Read the model definition and answer for the solid it produces. Units are mm, in the model's axes. Coordinates: 2 decimals unless noted, no trailing zeros. Write each loop counter-clockwise with the first axis right and the second up, starting at its lowest first coordinate (ties: lowest second). Pieces come first, ordered by that corner, then holes. Notation, with made-up numbers: (67.25, -20) -> (73.25, -20) arc R32 ccw to (73.25, 7) -> close; hole circle Ø11 at (-1.5, 9.25). An arc over 180 degrees is marked (long way). One line per item, written item: value. Start each with the question number.
1. Find section C-C, the plane y = 41.5. Write down the section's boundary in (x, z) (3 decimals).
2. Find section A-A, the plane y = -15.5. Write down the section's boundary in (x, z), and give its area (3 significant figures).
3. Given P1, Ø4, axis at x = -90, y = -41.5, coming from the -Z side, flat-ended and moving along its own axis, determine where the tip first touches the part or whether it passes through.
4. Consider line 1 along Y through (x, z) = (-90, 3.75) (3 decimals); line 2 along Y through (x, z) = (36, 6.75); line 3 along X through (y, z) = (21.5, 3.25). Determine where each line is inside the solid, lowest interval first.
5. Find section D-D, the plane z = 5.75. State how many separate pieces and enclosed holes the cut face has, and give its area (3 significant figures).
6. Find section B-B, the plane x = -71. Write down the section's boundary in (y, z), and give its area (3 significant figures).
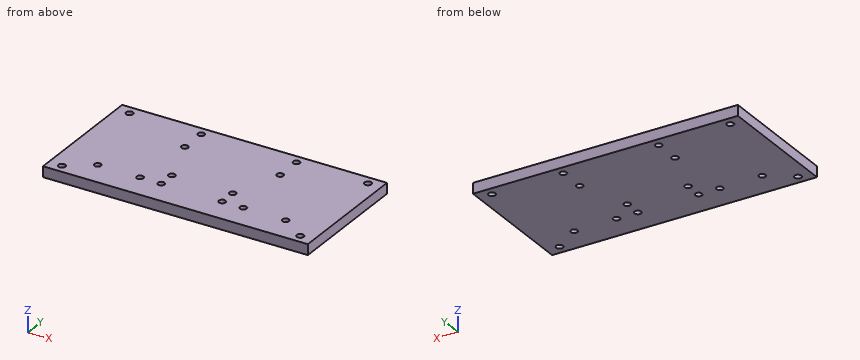
```python
from build123d import *

# Parameters (mm, degrees)
SKETCH_W   = 97
SKETCH_H   = 200
SKETCH_R   = 2.5
SKETCH_R_2 = 2.625
PAD_DEPTH  = 8


with BuildPart() as part:
    # Sketch → Pad (new body)
    with BuildSketch(Plane(origin=(0, 0, 0), x_dir=(0, 1, 0), z_dir=(0, 0, 1))):
        Rectangle(SKETCH_W, SKETCH_H)
        with Locations((-28.5, 71)):
            Circle(SKETCH_R, mode=Mode.SUBTRACT)
        with Locations((-28.5, 39)):
            Circle(SKETCH_R, mode=Mode.SUBTRACT)
        with Locations((-28.5, -39)):
            Circle(SKETCH_R, mode=Mode.SUBTRACT)
        with Locations((-28.5, -71)):
            Circle(SKETCH_R, mode=Mode.SUBTRACT)
        with Locations((-28.5, 23)):
            Circle(SKETCH_R, mode=Mode.SUBTRACT)
        with Locations((-15.5, 23)):
            Circle(SKETCH_R, mode=Mode.SUBTRACT)
        with Locations((-28.5, -23)):
            Circle(SKETCH_R, mode=Mode.SUBTRACT)
        with Locations((-15.5, -23)):
            Circle(SKETCH_R, mode=Mode.SUBTRACT)
        with Locations((-41.5, 90)):
            Circle(SKETCH_R_2, mode=Mode.SUBTRACT)
        with Locations((41.5, 90)):
            Circle(SKETCH_R_2, mode=Mode.SUBTRACT)
        with Locations((-41.5, -90)):
            Circle(SKETCH_R_2, mode=Mode.SUBTRACT)
        with Locations((41.5, -90)):
            Circle(SKETCH_R_2, mode=Mode.SUBTRACT)
        with Locations((21.5, 36)):
            Circle(SKETCH_R, mode=Mode.SUBTRACT)
        with Locations((41.5, 36)):
            Circle(SKETCH_R, mode=Mode.SUBTRACT)
        with Locations((21.5, -36)):
            Circle(SKETCH_R, mode=Mode.SUBTRACT)
        with Locations((41.5, -36)):
            Circle(SKETCH_R, mode=Mode.SUBTRACT)
    extrude(amount=PAD_DEPTH)


solid = part.part
```
Answer block:
1. outline: (-100, 0) -> (-92.625, 0) -> (-92.625, 8) -> (-100, 8) -> close; (-87.375, 0) -> (-38.5, 0) -> (-38.5, 8) -> (-87.375, 8) -> close; (-33.5, 0) -> (33.5, 0) -> (33.5, 8) -> (-33.5, 8) -> close; (38.5, 0) -> (87.375, 0) -> (87.375, 8) -> (38.5, 8) -> close; (92.625, 0) -> (100, 0) -> (100, 8) -> (92.625, 8) -> close
2. outline: (-100, 0) -> (-25.5, 0) -> (-25.5, 8) -> (-100, 8) -> close; (-20.5, 0) -> (20.5, 0) -> (20.5, 8) -> (-20.5, 8) -> close; (25.5, 0) -> (100, 0) -> (100, 8) -> (25.5, 8) -> close
2. area: 1,520 mm2
3. P1: passes through
4. line 1: y = -48.5 to -44.125, -38.875 to 38.875, 44.125 to 48.5
4. line 2: y = -48.5 to 19, 24 to 39, 44 to 48.5
4. line 3: x = -100 to -38.5, -33.5 to 33.5, 38.5 to 100
5. separate pieces: 1
5. enclosed holes: 16
5. area: 19,100 mm2
6. outline: (-48.5, 0) -> (-31, 0) -> (-31, 8) -> (-48.5, 8) -> close; (-26, 0) -> (48.5, 0) -> (48.5, 8) -> (-26, 8) -> close
6. area: 736 mm2
